Work out the finished part from the listing and answer in its coordinate system (mm). Coordinates: 2 decimals unless noted, no trailing zeros. Order: outer loops, then holes, each group sorted by start corner. A loop starts at its lowest first (then second) coordinate and runs counter-clockwise, first axis right, second up. Notation, with made-up numbers: M -28,39 L -1,39 A12 ccw -1,58 Z; hole C 60,61 d6. An arc over 180 degrees is marked long. Write item = value, one per line. Start each with the question number.
Q1. Determine the mould class of faces 1 (the flat face through (303.792, -0.028, -117.675)), 2 (the flat face through (241, 2, -11)), 3 (the flat face through (280.632, -0.028, -110.745)) for opening direction Z: released by +Z, released by -Z, zero draft, split by the parting line, or undercut.
Q2. Find section C-C on x = 374. Give the vertices of the cut face in (y, z).
Q3. Straight lines are drawn through the part: line 1 along Z through (x, y) = (60.5, -1.55); line 2 along Z through (x, y) = (429, -0.6); line 3 along X through (y, z) = (0.85, -164). For each, find the intervals that lie inside material, in ascending order.
Q4. Find section B-B on z = -122.5. Give the vertices of the cut face in (x, y), and give its area (3 significant figures).
Q5. Find section A-A on y = -0.2. Give the vertices of the cut face in (x, z).
Q6. Each of these flat-tipped pins is pushed along its axis until it touches: P1, Ø1, axis at x = 300, y = -0.5, coming from the +Z side; P2, Ø1.2, axis at x = 622.5, y = 1, coming from the -Z side; P3, Ø2, axis at y = 0.5, z = -57.5, coming from the +X side. Where does it stop, or does it pass through?
```python
from build123d import *

# Parameters (mm, degrees)
F1_DEPTH    = 2
F2_DEPTH    = 2
F3_DEPTH    = 2
F4_DEPTH    = 2
F5_T1_DEPTH = 4
F6_R        = 6.5


# Not quite as in the source:
# - a fillet or chamfer that OpenCascade refuses, or shapes differently, is made with other operations: its cross-section is extruded or revolved along the edge and cut away or added


with BuildPart() as f1:
    # F0 (on Front) → F1 (new body)
    with BuildSketch(Plane.XZ):
        Polygon((611.2015247345, 21.8497800332), (0, 0), (0, -250), (617.4515247345, 18.9482106362), (611.2015247345, 18.9482106362), align=None)
        Polygon((27.5068562478, -214.647129178), (27.5068562478, -19.3058601132), (526.7680287361, -9.7110727802), align=None, mode=Mode.SUBTRACT)
    extrude(amount=F1_DEPTH)

    # F0 (on Front) → F2 (join)
    with BuildSketch(Plane.XZ):
        Polygon((611.2015247345, 21.8497800332), (0, 0), (0, -250), (617.4515247345, 18.9482106362), (611.2015247345, 18.9482106362), align=None)
        Polygon((27.5068562478, -214.647129178), (27.5068562478, -19.3058601132), (526.7680287361, -9.7110727802), align=None, mode=Mode.SUBTRACT)
    extrude(amount=-F2_DEPTH)

    # F0 (on Front) → F3 (join)
    with BuildSketch(Plane.XZ):
        Polygon((611.2015247345, 23.9482106362), (611.2015247345, 21.8497800332), (611.2015247345, 18.9482106362), (617.4515247345, 18.9482106362), (623.7015247345, 18.9482106362), (623.7015247345, 23.9482106362), align=None)
    extrude(amount=F3_DEPTH)

    # F0 (on Front) → F4 (join)
    with BuildSketch(Plane.XZ):
        Polygon((611.2015247345, 23.9482106362), (611.2015247345, 21.8497800332), (611.2015247345, 18.9482106362), (617.4515247345, 18.9482106362), (623.7015247345, 18.9482106362), (623.7015247345, 23.9482106362), align=None)
    extrude(amount=-F4_DEPTH)

    # F5: fillet of radius 5 on 1 edges, made by hand

    # F5_s2 → F5_t1 (join)
    with BuildSketch(Plane.XZ.offset(-2)):
        with BuildLine():
            ThreePointArc((611.2015247345, 23.9482106362), (609.476442407, 22.3435494733), (607.20803479, 21.7070171746))
            Line((607.20803479, 21.7070171746), (611.2015247345, 21.8497800332))
            Line((611.2015247345, 21.8497800332), (611.2015247345, 23.9482106362))
        make_face()
    extrude(amount=F5_T1_DEPTH)

    # F6
    f6_edges = [f1.edges().sort_by_distance(p)[0] for p in [
        (617.451525, 0, 18.948211),
    ]]
    fillet(f6_edges, radius=F6_R)


solid = f1.part
```
Findings below:
q1.face_1 = released by -Z
q1.face_2 = zero draft
q1.face_3 = undercut
q2.outline = M -2,-87.09 L 2,-87.09 L 2,-72.42 L -2,-72.42 Z; M -2,-12.65 L 2,-12.65 L 2,13.37 L -2,13.37 Z
q3.line_1 = -223.65 to -201.1, -18.67 to 2.16
q3.line_2 = -63.14 to -49.84, -11.59 to 15.34
q3.line_3 = 0 to 27.51, 150.89 to 197.44
q4.outline = M 0,-2 L 27.51,-2 L 27.51,2 L 0,2 Z; M 251.99,-2 L 292.71,-2 L 292.71,2 L 251.99,2 Z
q4.area = 273 mm^2
q5.outline = M 0,-250 L 616.21,18.41 A6.5 cw 618.81,18.95 L 623.7,18.95 L 623.7,23.95 L 611.2,23.95 A5 cw 607.21,21.71 L 0,0 Z; hole M 27.51,-214.65 L 526.77,-9.71 L 27.51,-19.31 Z
q6.P1 = 10.74
q6.P2 = 18.95
q6.P3 = 444.24
